from build123d import *

# Parameters (mm, degrees)
ESQUISSE1_W             = 165
ESQUISSE1_H             = 150
BOSS_EXTRU_1_DEPTH      = 1.5
ESQUISSE2_R             = 1.5
ESQUISSE2_R_2           = 8
ESQUISSE2_R_3           = 4
ESQUISSE2_R_4           = 8.5
ENL_V_MAT_EXTRU_1_DEPTH = 182.251896542


with BuildPart() as part:
    # Esquisse1 → Boss.-Extru.1 (new body)
    with BuildSketch(Plane.XY):
        with Locations((82.5, 0)):
            Rectangle(ESQUISSE1_W, ESQUISSE1_H)
    extrude(amount=BOSS_EXTRU_1_DEPTH)

    # Esquisse2 → Enlèv. mat.-Extru.1 (cut, through all)
    with BuildSketch(Plane.XY.offset(1.5)):
        with Locations((158.25, 55)):
            Circle(ESQUISSE2_R)
        with Locations((158.25, -55)):
            Circle(ESQUISSE2_R)
        with Locations((151.25, 34.5)):
            Circle(ESQUISSE2_R)
        with Locations((83, -19)):
            Circle(ESQUISSE2_R)
        with Locations((143, -21)):
            Circle(ESQUISSE2_R)
        with Locations((15, 0)):
            Circle(ESQUISSE2_R_2)
        with Locations((15, 65)):
            Circle(ESQUISSE2_R_3)
        with Locations((15, -65)):
            Circle(ESQUISSE2_R_3)
        with Locations((50, 60)):
            Circle(ESQUISSE2_R_4)
        with Locations((68.75, 34.5)):
            Circle(ESQUISSE2_R)
        with Locations((68.75, -70)):
            Circle(ESQUISSE2_R)
        with BuildLine():
            Line((90, 10), (165, 10))
            ThreePointArc((165, 10), (179, -4), (165, -18))
            Line((165, -18), (90, -18))
            ThreePointArc((90, -18), (76, -4), (90, 10))
        make_face()
    extrude(amount=-ENL_V_MAT_EXTRU_1_DEPTH, mode=Mode.SUBTRACT)


solid = part.part
The model under review builds one solid part; all positions refer to its coordinate system, in mm. Round coordinates to 2 decimals unless told otherwise and drop trailing zeros. Loops run counter-clockwise (first coordinate to the right, second up) from the corner with the lowest first, then second, coordinate; pieces in that order, holes last. Notation, with made-up numbers: (53, 52) - (112, 52) arc R14 ccw to (112, 78) - close; hole circle Ø7 at (4.5, -26.5). An arc over 180 degrees is marked (long way). Use CSV: the item, a comma, the result in double quotes.
(1) Take a section at A-A, the plane x = 112. Give the boundary of the cut face in (y, z).
Working result:
outline,"(-75, 0) - (-18, 0) - (-18, 1.5) - (-75, 1.5) - close; (10, 0) - (75, 0) - (75, 1.5) - (10, 1.5) - close"
(2) For line 1 (Y direction, x = 68.75, z = 1.2); line 2 (Y direction, x = 151, z = 0.65); line 3 (Y direction, x = 15, z = 0.4), list the stretches that pass through material, from the lowest coordinate up.
Working result:
line 1,"y = -75 to -71.5, -68.5 to 33, 36 to 75"
line 2,"y = -75 to -18, 10 to 33.02, 35.98 to 75"
line 3,"y = -75 to -69, -61 to -8, 8 to 61, 69 to 75"
(3) The part is to be moulded in two halves that separate along Y. For faces 1 (the cylindrical face through (48.16, 51.7, 0.76)), 2 (the flat face through (63, 1, 0)), say which applies: pulls with the +Y half, pulls with the -Y half, needs draft (parallel to the pull), parting line crosses it, or undercut.
Working result:
face 1,"undercut"
face 2,"needs draft"
(4) Take a section at D-D, the plane y = 0. Give the boundary of the cut face in (x, z).
Working result:
outline,"(0, 0) - (7, 0) - (7, 1.5) - (0, 1.5) - close; (23, 0) - (76.58, 0) - (76.58, 1.5) - (23, 1.5) - close"
(5) Clearance check with a flat-ended pin moving along its axis: P1, Ø2.5, axis at x = 143, y = -21, coming from the +Z side. State where the tip first meets the part, or that it passes through.
Working result:
P1,"passes through"
(6) Take a section at C-C, the plane x = 15. Give the boundary of the cut face in (y, z).
Working result:
outline,"(-75, 0) - (-69, 0) - (-69, 1.5) - (-75, 1.5) - close; (-61, 0) - (-8, 0) - (-8, 1.5) - (-61, 1.5) - close; (8, 0) - (61, 0) - (61, 1.5) - (8, 1.5) - close; (69, 0) - (75, 0) - (75, 1.5) - (69, 1.5) - close"
(7) Take a section at B-B, the plane z = 0.45. State how many separate pieces and enclosed holes the cut face has, plus the area to 3 significant figures.
Working result:
separate pieces,"1"
enclosed holes,"11"
area,"21,800 mm^2"
